Can you work these out from the drawing? Everything is in mm from the part's minimum corner. A direction names the side the tool comes from. Give positions to 0.01 mm unless a question says otherwise; leave off trailing zeros. Loops run counter-clockwise (first coordinate to the right, second up) from the corner with the lowest first, then second, coordinate; pieces in that order, holes last. Notation, with made-up numbers: (17, -31) -> (72, -31) arc R8 ccw to (72, -17) -> close; hole circle Ø4 at (-32, -17). An arc over 180 degrees is marked (long way). Return JSON: item names as keys, results as strings. Group by question number.
Q1. Suppose I cut it at B-B, the plane x = 38. Please give me the cut outline in (y, z), and give its area (3 significant figures).
Q2. I need wall thicknesses on line 1 along Y through (x, z) = (40.5, 7.5); line 2 along X through (y, z) = (8.5, 22.5); line 3 along X through (y, z) = (24, 7) (1 decimal). Which ranges of each line are inside material? Lowest first, please. Write a range as [from, to].
Q3. Will these pins go through, and if not, where does the flat tip stop? pin 1 (4 mm diameter, centred on x = 31.5, z = 23, fed in from +Y); pin 2 (8 mm diameter, centred on y = 32, z = 28, fed in from +X); pin 3 (1 mm diameter, centred on y = 11, z = 18.5, fed in from +X).
Q4. Suppose I cut it at D-D, the plane z = 23. Please give me the cut outline in (x, y).
Q5. Suppose I cut it at C-C, the plane y = 9. Please give me the cut outline in (x, z), and give its area (3 significant figures).
Q6. Suppose I cut it at A-A, the plane z = 3.5. Please give me the cut outline in (x, y), and give its area (3 significant figures).
Q7. Which directions (+Z, -Z, +X, -X, +Y, -Y) give clear straight access to the entire face, cutting with the end or side of a thin tool? Please do the marked faces 1, 2 and 3.
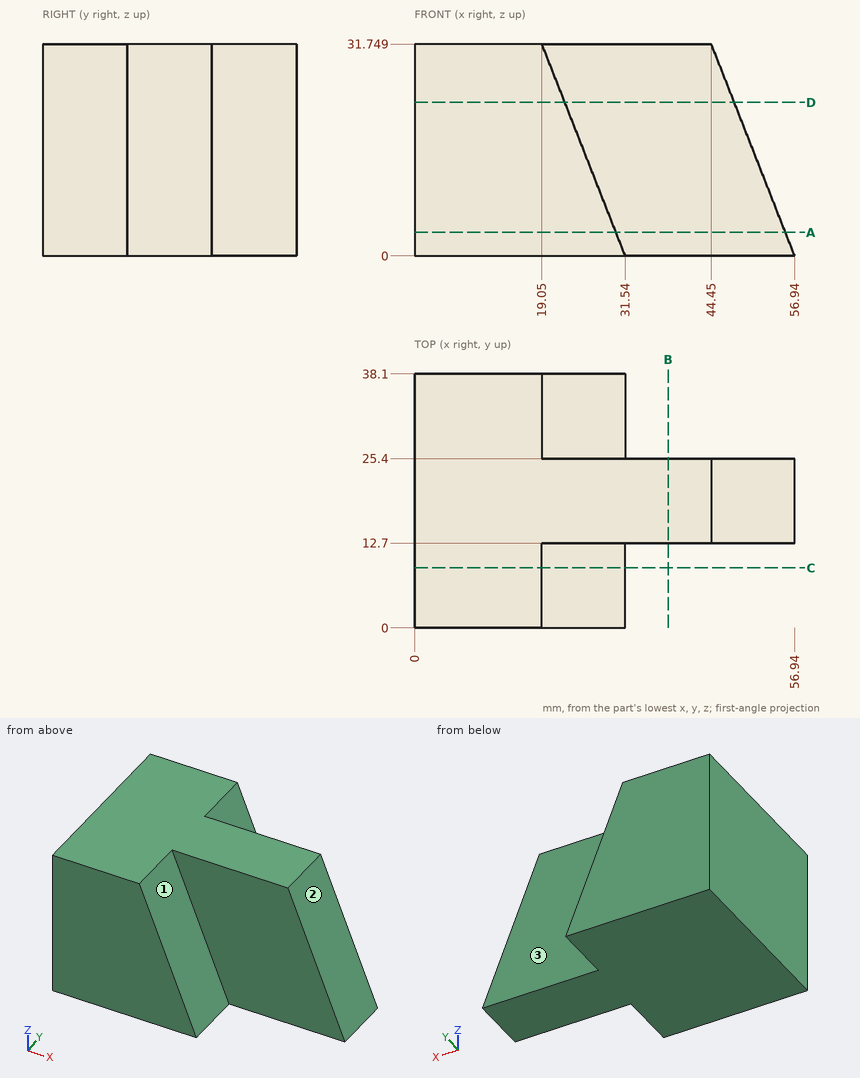
Ans:
{
 "1": {"outline": "(12.7, 0) -> (25.4, 0) -> (25.4, 31.75) -> (12.7, 31.75) -> close", "area": "403 mm^2"},
 "2": {"line 1": "y = [12.7, 25.4]", "line 2": "x = [0, 22.69]", "line 3": "x = [0, 54.2]"},
 "3": {"pin 1": "stops at y = 25.4", "pin 2": "stops at x = 22.1", "pin 3": "stops at x = 24.46"},
 "4": {"outline": "(0, 0) -> (22.49, 0) -> (22.49, 12.7) -> (47.89, 12.7) -> (47.89, 25.4) -> (22.49, 25.4) -> (22.49, 38.1) -> (0, 38.1) -> close"},
 "5": {"outline": "(0, 0) -> (31.54, 0) -> (19.05, 31.75) -> (0, 31.75) -> close", "area": "803 mm^2"},
 "6": {"outline": "(0, 0) -> (30.16, 0) -> (30.16, 12.7) -> (55.56, 12.7) -> (55.56, 25.4) -> (30.16, 25.4) -> (30.16, 38.1) -> (0, 38.1) -> close", "area": "1,470 mm^2"},
 "7": {"face 1": "+Z, +X, -Y", "face 2": "+Z, +X, +Y, -Y", "face 3": "+Z, +X, +Y"}
}
